Model file for the job. Use its own axes, mm. A direction names the side the tool comes from. Round coordinates to 2 decimals unless told otherwise and drop trailing zeros. Loops run counter-clockwise (first coordinate to the right, second up) from the corner with the lowest first, then second, coordinate; pieces in that order, holes last. Notation, with made-up numbers: M -1.75,-17.5 L 17.25,-17.5 A16 cw 17.25,-9.5 Z; hole C 31,-18.75 d8. An arc over 180 degrees is marked long. Use a Markdown table: item, result. Add a question column.
Item 1: Wall check: L1, parallel to X at y = 7, z = 9.75; L2, parallel to Z at x = -19, y = 15.5. Give the ranges that are in metal, low to high. Write a range as from..to.
Item 2: Saw through at C-C on z = 7. Write the cut outline in (x, y), then the cut area to 3 significant figures.
Item 3: Saw through at B-B on x = -2. Write the cut outline in (y, z), then the cut area to 3 significant figures.
Item 4: Tool access for faces 5 (the flat face through (-1, -38, 4)), 6 (the cylindrical face through (44.92, 0.58, 18.5)): list every direction of +Z, -Z, +X, -X, +Y, -Y with a clear straight run to the whole face (end or side of a thin tool).
Item 5: Two-plate mould, pull along Y, no slides. Class faces 1 (the cylindrical face through (0.58, 44.92, 18.5)), 2 (the flat face through (-1, 1, 20)), 3 (the flat face through (-1, 1, 15)), 4 (the flat face through (38, -1, 7)): +Y half, -Y half, draft (parallel to the pull), parting line (faces both ways), or undercut.
Item 6: Saw through at A-A on y = -20.5. Write the cut outline in (x, z), then the cut area to 3 significant figures.
```python
from build123d import *

# Parameters (mm, degrees)
F0_W     = 92.7
F0_H     = 92.7
F0_W_2   = 76
F0_H_2   = 76
F1_DEPTH = 20
F2_R     = 5
F4_DEPTH = 15
F5_DEPTH = 8.35


with BuildPart() as f1:
    # F0 (on Top) → F1 (new body)
    with BuildSketch(Plane.XY):
        Rectangle(F0_W, F0_H)
        Rectangle(F0_W_2, F0_H_2, mode=Mode.SUBTRACT)
        Rectangle(F0_W_2, F0_H_2)
    extrude(amount=F1_DEPTH)

    # F2
    f2_edges = [f1.edges().sort_by_distance(p)[0] for p in [
        (-46.35, 0, 20),
        (0, 46.35, 20),
        (46.35, 0, 20),
        (0, -46.35, 20),
        (46.35, -46.35, 10),
        (-46.35, -46.35, 10),
        (46.35, 46.35, 10),
        (-46.35, 46.35, 10),
    ]]
    fillet(f2_edges, radius=F2_R)

    # F0 (on Top) → F4 (cut)
    with BuildSketch(Plane.XY):
        Rectangle(F0_W_2, F0_H_2)
    extrude(amount=F4_DEPTH, mode=Mode.SUBTRACT)

    # F3 (on face) → F5 (cut, through all)
    with BuildSketch(Plane.XZ.offset(46.35)):
        with BuildLine():
            ThreePointArc((0, 15), (-5, 10), (0, 5))
            ThreePointArc((0, 5), (3.535534, 6.464466), (5, 10))
            ThreePointArc((5, 10), (3.535534, 13.535534), (0, 15))
        make_face()
    extrude(amount=-F5_DEPTH, mode=Mode.SUBTRACT)


solid = f1.part
```
Entries:
| question | item | result |
|---|---|---|
| 1 | L1 | -46.35..-38, 38..46.35 |
| 1 | L2 | 15..20 |
| 2 | outline | M -46.35,-41.35 A5 ccw -41.35,-46.35 L -4,-46.35 L -4,-38 L -38,-38 L -38,38 L 38,38 L 38,-38 L 4,-38 L 4,-46.35 L 41.35,-46.35 A5 ccw 46.35,-41.35 L 46.35,41.35 A5 ccw 41.35,46.35 L -41.35,46.35 A5 ccw -46.35,41.35 Z |
| 2 | area | 2,730 mm2 |
| 3 | outline | M -46.35,0 L -38,0 L -38,5.42 L -46.35,5.42 Z; M -46.35,14.58 L -38,14.58 L -38,15 L 38,15 L 38,0 L 46.35,0 L 46.35,15 A5 ccw 41.35,20 L -41.35,20 A5 ccw -46.35,15 Z |
| 3 | area | 627 mm2 |
| 4 | face 5 | -Z |
| 4 | face 6 | +Z, +X, +Y, -Y |
| 5 | face 1 | +Y half |
| 5 | face 2 | draft |
| 5 | face 3 | undercut |
| 5 | face 4 | undercut |
| 6 | outline | M -46.35,0 L -38,0 L -38,15 L 38,15 L 38,0 L 46.35,0 L 46.35,15 A5 ccw 41.35,20 L -41.35,20 A5 ccw -46.35,15 Z |
| 6 | area | 703 mm2 |
